from build123d import *

# Parameters (mm, degrees)
F1_DEPTH = 25.4
F2_W     = 25.4
F2_H     = 25.4
F3_DEPTH = 12.7


with BuildPart() as f1:
    # F0 (on Front) → F1 (new body)
    with BuildSketch(Plane.XZ):
        Polygon((0, 76.2), (0, 38.1), (71.701042, 38.1), (38.1, 76.2), align=None)
        Polygon((0, 25.4), (0, 0), (127, 0), (127, 38.1), (71.701042, 38.1), (0, 38.1), align=None)
    extrude(amount=F1_DEPTH)

    # F2 (on face) → F3 (join)
    with BuildSketch(Plane.XZ.offset(25.4)):
        with Locations((12.7, 12.7)):
            Rectangle(F2_W, F2_H)
    extrude(amount=F3_DEPTH)


solid = f1.part
Can you work these out from the model? Positions are in its coordinate system, mm. A direction names the side the tool comes from. Coordinates: 2 decimals unless noted, no trailing zeros. Write each loop counter-clockwise with the first axis right and the second up, starting at its lowest first coordinate (ties: lowest second). Pieces come first, ordered by that corner, then holes. Notation, with made-up numbers: (74, 87.25) -> (133, 87.25) arc R21 ccw to (133, 108.25) -> close; hole circle Ø5 at (22, -37.5). An arc over 180 degrees is marked (long way). Write item = value, one per line.
(1) Imagine slicing it at B-B (z = 9). Please give me the cut outline in (x, y), and give its area (3 significant figures).
Verdict:
outline = (0, -38.1) -> (25.4, -38.1) -> (25.4, -25.4) -> (127, -25.4) -> (127, 0) -> (0, 0) -> close
area = 3,550 mm^2
(2) For pin 1 (4 mm diameter, centred on x = 12.5, y = -33, fed in from +Z); pin 2 (1 mm diameter, centred on x = 40.5, y = -6, fed in from +Z); pin 3 (4 mm diameter, centred on y = -28.5, z = 8.5, fed in from +X), each with a flat end and sliding along its axis, tell me the tip position at first contact or that it passes through.
Verdict:
pin_1 = 25.4
pin_2 = 74.05
pin_3 = 25.4
(3) Imagine slicing it at C-C (x = 32.5). Please give me the cut outline in (y, z), and give its area (3 significant figures).
Verdict:
outline = (-25.4, 0) -> (0, 0) -> (0, 76.2) -> (-25.4, 76.2) -> close
area = 1,940 mm^2
(4) Imagine slicing it at D-D (z = 30.5). Please give me the cut outline in (x, y).
Verdict:
outline = (0, -25.4) -> (127, -25.4) -> (127, 0) -> (0, 0) -> close
(5) Imagine slicing it at A-A (x = 10). Please give me the cut outline in (y, z), and give its area (3 significant figures).
Verdict:
outline = (-38.1, 0) -> (0, 0) -> (0, 76.2) -> (-25.4, 76.2) -> (-25.4, 25.4) -> (-38.1, 25.4) -> close
area = 2,260 mm^2
(6) On a 3-axis mill with a long thin cutter (end or side, diameter ignored), from which of +Z, -Z, +X, -X, +Y, -Y can I reach the whole of each face in a straight line? I mean faces 1 (the face through (13, -32, 25.4)), 2 (the face through (100, -13, 38.1)), 3 (the face through (25.4, -32, 13)), 4 (the face through (63, -15, 0)). Say none if no direction works.
Verdict:
face_1 = +Z, +X, -X, -Y
face_2 = +Z, +X, +Y, -Y
face_3 = +Z, -Z, +X, -Y
face_4 = -Z, +X, -X, +Y, -Y
(7) If I drill on probe 1 along Y at (x, z) = (63, 46.5); probe 2 along Z at (x, y) = (112, -22.5); probe 3 along X at (y, z) = (-36, 13), over which ranges is the centre line in solid material (lowest first)?
Verdict:
probe_1 = -25.4 to 0
probe_2 = 0 to 38.1
probe_3 = 0 to 25.4
